The listing builds one solid part. Answer for the finished solid, in the listing's coordinates (mm). A direction names the side the tool comes from. Give positions to 0.01 mm unless a question says otherwise; leave off trailing zeros. Write each loop counter-clockwise with the first axis right and the second up, starting at its lowest first coordinate (ties: lowest second). Pieces come first, ordered by that corner, then holes. Notation, with made-up numbers: M 10,-22 L 28,-22 A15 ccw 28,2 Z; hole C 60.25,23.5 d10. An arc over 180 degrees is marked long. Return JSON: item names as keys, results as strings.
from build123d import *

# Parameters (mm, degrees)
F0_R     = 152.4
F3_DEPTH = 57.15
F4_DEPTH = 57.15


with BuildPart() as f2:
    # F2: sweep along a path in F1
    with BuildLine(Plane.XY) as f2_path:
        ThreePointArc((-323.2892203585, 323.2892203585), (-422.3977222642, 174.9628652773), (-457.2, 0))
    # F0 (on Front) → F2 (sweep)
    with BuildSketch(Plane.XZ):
        with Locations((-457.2, 0)):
            Circle(F0_R)
    sweep(path=f2_path.line)

    # F3 (add): a face of the model
    f3_faces = [f2.faces().sort_by_distance(p)[0] for p in [
        (-457.2, 0, 0),
    ]]
    extrude(f3_faces, amount=F3_DEPTH)

    # F4 (add): a face of the model
    f4_faces = [f2.faces().sort_by_distance(p)[0] for p in [
        (-323.2892203585, 323.2892203585, 0),
    ]]
    extrude(f4_faces, amount=F4_DEPTH)


solid = f2.part
Item 1: A cutting plane is placed at B-B, the plane z = -55. Write down the section's boundary in (x, y), plus the area to 3 significant figures.
Geometry results:
{"outline": "M -599.33,-57.15 L -315.07,-57.15 L -315.07,0 A315.07 cw -222.79,222.79 L -182.38,263.2 L -383.38,464.2 L -423.79,423.79 A599.33 ccw -599.33,0 Z", "area": "135,000 mm2"}
Item 2: A cutting plane is placed at A-A, the plane z = 0. Write down the section's boundary in (x, y) (3 decimals).
Geometry results:
{"outline": "M -609.6,-57.15 L -304.8,-57.15 L -304.8,0 A304.8 cw -215.526,215.526 L -175.115,255.937 L -390.641,471.463 L -431.052,431.052 A609.6 ccw -609.6,0 Z"}
Item 3: Find the intervals of material crossed by line 1 (Z direction, x = -375.5, y = 261); line 2 (Z direction, x = -316, y = 14); line 3 (X direction, y = 431.5, z = 86), in increasing order.
Geometry results:
{"line 1": "z = -152.4 to 152.4", "line 2": "z = -58.1 to 58.1", "line 3": "x = -393.01 to -350.68"}
Item 4: Given pin 1 Ø12 at (y, z) = (227, -37) entering from +X; pin 2 Ø12 at (x, y) = (-532.5, 4) entering from -Z; pin 3 Ø2 at (x, y) = (-308.5, 217) entering from -Z, each flat-ended and moving along its own axis, determine where each tip first touches the part or whether it passes through.
Geometry results:
{"pin 1": "stops at x = -204.16", "pin 2": "stops at z = -135.72", "pin 3": "stops at z = -130.31"}
Item 5: Which of the six approach directions +Z, -Z, +X, -X, +Y, -Y give full straight-line access (tool end or side, diameter ignored) to faces 1 (the cylindrical face through (-311.84, -28.17, -45.78)), 2 (the flat face through (-284.39, 365.21, 2.13))?
Geometry results:
{"face 1": "-Y", "face 2": "+Z, -Z, +X, +Y"}
